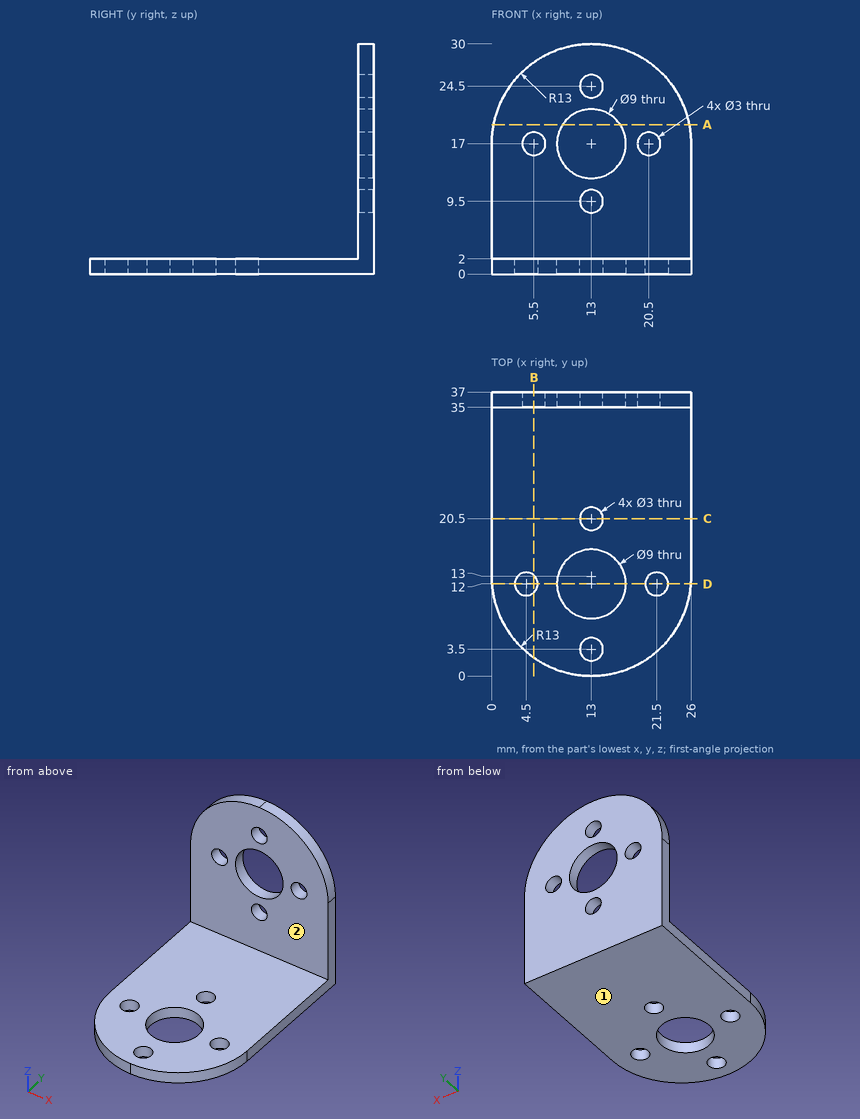
For this review, use the dimensioned drawing (mm, ordinates from the lowest corner) and the shaded views. A direction names the side the tool comes from. Coordinates: 2 decimals unless noted, no trailing zeros. Loops run counter-clockwise (first coordinate to the right, second up) from the corner with the lowest first, then second, coordinate; pieces in that order, holes last.
1. Add section A-A, the plane z = 19.5. Give the boundary of the cut face in (x, y), then the cut area to 3 significant figures.
2. Add section D-D, the plane y = 12. Give the boundary of the cut face in (x, z), then the cut area to 3 significant figures.
3. For the marked faces 1 and 2, list the 3-axis set-ups (+Z, -Z, +X, -X, +Y, -Y) from which the entire face can be reached by the end or side of a thin tool; tool diameter is ignored.
4. Add section B-B, the plane x = 5.5. Give the boundary of the cut face in (y, z).
5. For line 1 (Y direction, x = 8.5, z = 8); line 2 (Z direction, x = 1.75, y = 19); line 3 (Y direction, x = 21.5, z = 1.5), list the stretches that pass through material, from the lowest coordinate up.
6. Insertion check: P1, Ø3.5, axis at x = 13, y = 3.5, coming from the +Z side; P2, Ø8, axis at x = 12.5, z = 14.5, coming from the -Y side. Each pin has a flat end and moves straight along its axis. Give the tip position at first contact, or say it passes through.
7. Add section C-C, the plane y = 20.5. Give the boundary of the cut face in (x, z).
Result:
1. outline: (0.24, 35) - (9.26, 35) - (9.26, 37) - (0.24, 37) - close; (16.74, 35) - (25.76, 35) - (25.76, 37) - (16.74, 37) - close
1. area: 36.1 mm2
2. outline: (0.04, 0) - (3, 0) - (3, 2) - (0.04, 2) - close; (6, 0) - (8.5, 0) - (8.5, 2) - (6, 2) - close; (17.5, 0) - (20, 0) - (20, 2) - (17.5, 2) - close; (23, 0) - (25.96, 0) - (25.96, 2) - (23, 2) - close
2. area: 21.8 mm2
3. face 1: -Z, +X, -X, +Y, -Y
3. face 2: +Z, +X, -X, -Y
4. outline: (2.38, 0) - (10.88, 0) - (10.88, 2) - (2.38, 2) - close; (13.12, 0) - (37, 0) - (37, 15.5) - (35, 15.5) - (35, 2) - (13.12, 2) - close; (35, 18.5) - (37, 18.5) - (37, 27.62) - (35, 27.62) - close
5. line 1: y = 35 to 37
5. line 2: z = 0 to 2
5. line 3: y = 3.16 to 10.5, 13.5 to 37
6. P1: stops at z = 2
6. P2: stops at y = 35
7. outline: (0, 0) - (11.5, 0) - (11.5, 2) - (0, 2) - close; (14.5, 0) - (26, 0) - (26, 2) - (14.5, 2) - close
